from build123d import *

# Parameters (mm, degrees)
SKETCH1_W           = 152.4
SKETCH1_H           = 152.4
BOSS_EXTRUDE1_DEPTH = 12.7
SKETCH2_W           = 12.7
SKETCH2_H           = 25.4
BOSS_EXTRUDE2_DEPTH = 25.4
FILLET1_RADIUS      = 6.35
FILLET1_LENGTH      = 50.8
SKETCH3_W           = 38.1
SKETCH3_H           = 35.536125939
CUT_EXTRUDE1_DEPTH  = 50.8
SKETCH4_R           = 3.81
CUT_EXTRUDE2_DEPTH  = 50.8
SKETCH11_W          = 19.05
SKETCH11_H          = 30.48
BOSS_EXTRUDE6_DEPTH = 76.2
SKETCH14_R          = 12.7
CUT_EXTRUDE3_DEPTH  = 76.2
SKETCH14_3_R        = 12.7
CUT_EXTRUDE4_DEPTH  = 10.16


with BuildPart() as part:
    # Sketch1 → Boss-Extrude1 (new body)
    with BuildSketch(Plane(origin=(0, 0, 0), x_dir=(1, 0, 0), z_dir=(0, 1, 0))):
        Rectangle(SKETCH1_W, SKETCH1_H)
    extrude(amount=BOSS_EXTRUDE1_DEPTH)

    # Sketch2 → Boss-Extrude2 (add, symmetric)
    with BuildSketch(Plane(origin=(0, 0, 0), x_dir=(0, 0, -1), z_dir=(1, 0, 0))):
        with Locations((-57.15, 25.4)):
            Rectangle(SKETCH2_W, SKETCH2_H)
    extrude(amount=BOSS_EXTRUDE2_DEPTH, both=True)

    # Fillet1: full round fillet: the end face becomes a half cylinder, R = half its width
    fillet1_face = Plane((0, 38.1, 57.15), x_dir=(1, 0, 0), z_dir=(0, 1, 0))  # on the end face: x along it, z out of the body
    fillet1_slab = fillet1_face.offset(-FILLET1_RADIUS / 2) * Box(FILLET1_LENGTH, 2 * FILLET1_RADIUS, FILLET1_RADIUS, mode=Mode.PRIVATE)  # the body's end, R deep
    fillet1_round = Plane((0, 31.75, 57.15), x_dir=(0, 1, 0), z_dir=(1, 0, 0)) * Cylinder(FILLET1_RADIUS, FILLET1_LENGTH, mode=Mode.PRIVATE)  # its axis R under the face
    add(fillet1_slab - fillet1_round, mode=Mode.SUBTRACT)

    # Sketch3 → Cut-Extrude1 (cut)
    with BuildSketch(Plane.XY.offset(63.5)):
        with Locations((0, 30.46806297)):
            Rectangle(SKETCH3_W, SKETCH3_H)
    extrude(amount=-CUT_EXTRUDE1_DEPTH, mode=Mode.SUBTRACT)

    # Sketch4 → Cut-Extrude2 (cut)
    with BuildSketch(Plane(origin=(25.4, 0, 0), x_dir=(0, 0, -1), z_dir=(1, 0, 0))):
        with Locations((-57.15, 31.75)):
            Circle(SKETCH4_R)
    extrude(amount=-CUT_EXTRUDE2_DEPTH, mode=Mode.SUBTRACT)

    # Sketch11 → Boss-Extrude6 (add)
    with BuildSketch(Plane.XZ):
        with Locations((-9.525, -17.78)):
            Rectangle(SKETCH11_W, SKETCH11_H)
        with Locations((9.525, -17.78)):
            Rectangle(SKETCH11_W, SKETCH11_H)
        with Locations((9.525, 12.7)):
            Rectangle(SKETCH11_W, SKETCH11_H)
        with Locations((-9.525, 12.7)):
            Rectangle(SKETCH11_W, SKETCH11_H)
    extrude(amount=BOSS_EXTRUDE6_DEPTH)

    # Sketch14 → Cut-Extrude3 (cut)
    with BuildSketch(Plane(origin=(0, 12.7, 0), x_dir=(1, 0, 0), z_dir=(0, 1, 0))):
        with Locations(Location((0, 17.78, 0), (0, 0, 270))):
            Circle(SKETCH14_R)
        with Locations(Location((0, -12.7, 0), (0, 0, 270))):
            Circle(SKETCH14_R)
    extrude(amount=-CUT_EXTRUDE3_DEPTH, mode=Mode.SUBTRACT)

    # Sketch14<3> → Cut-Extrude4 (cut)
    with BuildSketch(Plane(origin=(0, 12.7, 0), x_dir=(1, 0, 0), z_dir=(0, 1, 0))):
        with Locations(Location((0, 48.26, 0), (0, 0, 270))):
            Circle(SKETCH14_3_R)
    extrude(amount=-CUT_EXTRUDE4_DEPTH, mode=Mode.SUBTRACT)


solid = part.part
Could you check a few things on this model? Use its own coordinates, in mm. A direction names the side the tool comes from. Coordinates: 2 decimals unless noted, no trailing zeros. Write each loop counter-clockwise with the first axis right and the second up, starting at its lowest first coordinate (ties: lowest second). Pieces come first, ordered by that corner, then holes. Notation, with made-up numbers: (-38, -28.5) - (1, -28.5) arc R29 cw to (1, 1.5) - close; hole circle Ø6 at (50, -8). An arc over 180 degrees is marked (long way). Write item = value, one per line.
1) We'd pull the mould along Z, two halves only. Please class faces 1 (the cylindrical face through (22.27, 30.29, 53.63)), 2 (the flat face through (76.2, 6, 1)), 3 (the cylindrical face through (-22.2, 38.1, 57)): +Z half, -Z half, draft (parallel to the pull), parting line (faces both ways), or undercut.
Result set:
face_1 = undercut
face_2 = draft
face_3 = parting line
2) Suppose I cut it at A-A on z = 57.15. Please give me the cut outline in (x, y), plus the area to 3 significant figures.
Result set:
outline = (-76.2, 0) - (76.2, 0) - (76.2, 12.7) - (25.4, 12.7) - (25.4, 27.94) - (19.05, 27.94) - (19.05, 12.7) - (-19.05, 12.7) - (-19.05, 27.94) - (-25.4, 27.94) - (-25.4, 12.7) - (-76.2, 12.7) - close; (-25.4, 35.56) - (-19.05, 35.56) - (-19.05, 38.1) - (-25.4, 38.1) - close; (19.05, 35.56) - (25.4, 35.56) - (25.4, 38.1) - (19.05, 38.1) - close
area = 2,160 mm2
3) Suppose I cut it at B-B on y = 16. Please give me the cut outline in (x, z).
Result set:
outline = (-25.4, 50.8) - (-19.05, 50.8) - (-19.05, 63.5) - (-25.4, 63.5) - close; (19.05, 50.8) - (25.4, 50.8) - (25.4, 63.5) - (19.05, 63.5) - close
4) Suppose I cut it at C-C on x = 0. Please give me the cut outline in (y, z).
Result set:
outline = (-76.2, -33.02) - (0, -33.02) - (0, -76.2) - (12.7, -76.2) - (12.7, -60.96) - (2.54, -60.96) - (2.54, -35.56) - (12.7, -35.56) - (12.7, -30.48) - (-63.5, -30.48) - (-63.5, -5.08) - (12.7, -5.08) - (12.7, 0) - (-63.5, 0) - (-63.5, 25.4) - (12.7, 25.4) - (12.7, 76.2) - (0, 76.2) - (0, 27.94) - (-76.2, 27.94) - close
5) For faces 4 (the cylindrical face through (3.815, -24.867, 24.814)), 5 (the flat face through (19.05, 22, 57)), 6 (the flat face through (-22, 22, 63.5)), which set-ups out of +Z, -Z, +X, -X, +Y, -Y let a thin tool reach every point of the face, with its end or its side?
Result set:
face_4 = +Y
face_5 = +Z, -Z, +Y
face_6 = +Z, +X, -X, +Y
6) Please list where these lines run through material, in increasing order: line 1 (X direction, y = -38.5, z = 12.7); line 2 (Y direction, x = -20.75, z = 57.15); line 3 (Z direction, x = 3, y = -25). Write a range as [from, to].
Result set:
line_1 = [-19.05, -12.7], [12.7, 19.05]
line_2 = [0, 27.94], [35.56, 38.1]
line_3 = [-33.02, -30.12], [-5.44, 0.36], [25.04, 27.94]
7) Suppose I cut it at D-D on y = -52.5. Please give me the cut outline in (x, z), plus the area to 3 significant figures.
Result set:
outline = (-19.05, -33.02) - (19.05, -33.02) - (19.05, 27.94) - (-19.05, 27.94) - close; hole circle Ø25.4 at (0, -17.78); hole circle Ø25.4 at (0, 12.7)
area = 1,310 mm2
8) Will these pins go through, and if not, where does the flat tip stop? pin 1 Ø4 at (y, z) = (23.5, 55) entering from -X; pin 2 Ø3 at (y, z) = (-4, -14) entering from +X; pin 3 Ø12 at (x, y) = (18, -38.5) entering from +Z.
Result set:
pin_1 = -25.4
pin_2 = 19.05
pin_3 = 27.94
